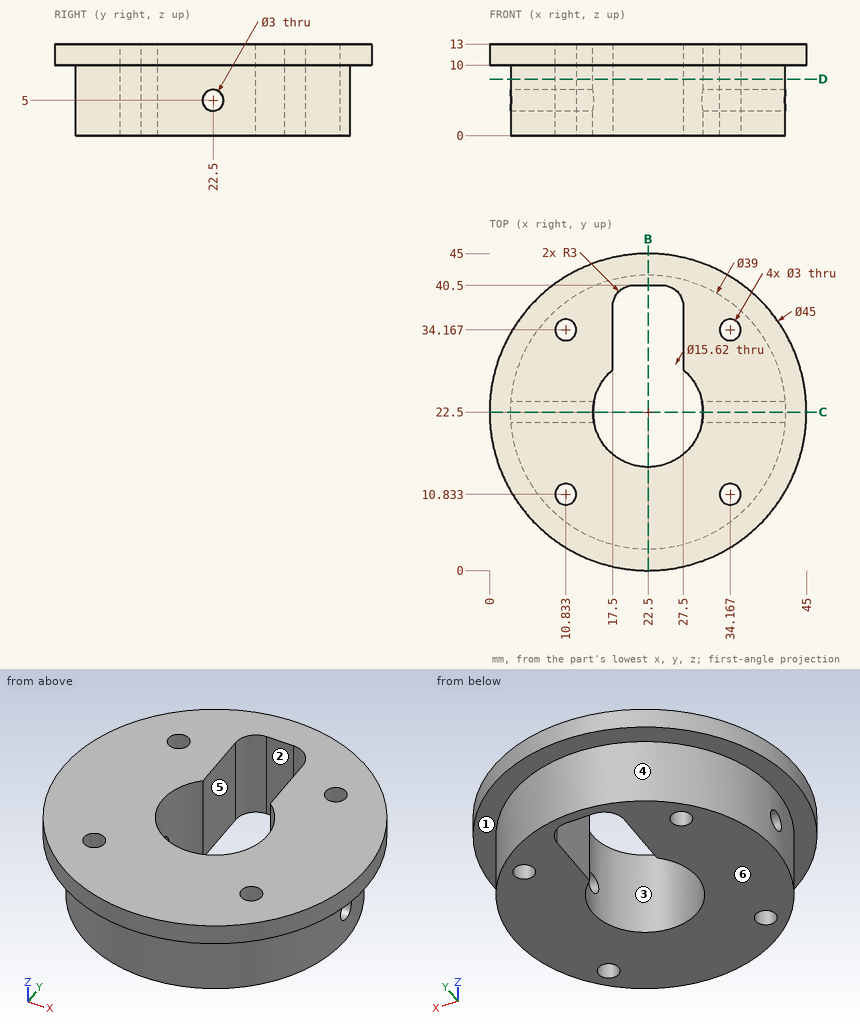
Can you work these out from the drawing? Everything is in mm from the part's minimum corner. A direction names the side the tool comes from. Give positions to 0.01 mm unless a question says otherwise; leave off trailing zeros. Order: outer loops, then holes, each group sorted by start corner. A loop starts at its lowest first (then second) coordinate and runs counter-clockwise, first axis right, second up. Notation, with made-up numbers: M 34,71.5 L 92,71.5 A26 ccw 92,99.5 Z; hole C -30.5,28 d8. An arc over 180 degrees is marked long. Use a Markdown table: item, result. Add a question column.
Item 1: If I drill on L1, parallel to Y at x = 35.5, z = 5.5 (1 decimal); L2, parallel to X at y = 22.5, z = 9; L3, parallel to X at y = 35.5, z = 6.5 (1 decimal), over which ranges is the centre line in solid material (lowest first)? Write a range as [from, to].
Item 2: Suppose I cut it at B-B (x = 22.5). List the corners of the cut face in (y, z) for me.
Item 3: For the marked faces 5 and 6, which set-ups out of +Z, -Z, +X, -X, +Y, -Y let a thin tool reach every point of the face, with its end or its side?
Item 4: We'd pull the mould along X, two halves only. Please class the marked faces 1, 2, 3 and 4: +X half, -X half, draft (parallel to the pull), parting line (faces both ways), or undercut.
Item 5: Suppose I cut it at D-D (z = 8). List the corners of the cut face in (x, y) for me, then the cut area to 3 significant figures.
Item 6: Suppose I cut it at C-C (y = 22.5). List the corners of the cut face in (x, z) for me, then the cut area to 3 significant figures.
Item 7: Will these pins go through, and if not, where does the flat tip stop? pin 1 (2.5 mm diameter, centred on y = 22.5, z = 5, fed in from +X); pin 2 (6 mm diameter, centred on x = 12, z = 6.5, fed in from -Y); pin 3 (4 mm diameter, centred on x = 21, z = 2, fed in from +Y); pin 4 (4.5 mm diameter, centred on y = 34.5, z = 8.5, fed in from +X).
Answer sheet:
| question | item | result |
|---|---|---|
| 1 | L1 | y = [8, 10.1], [11.5, 21.1], [23.9, 33.5], [34.9, 37] |
| 1 | L2 | x = [3, 14.69], [30.31, 42] |
| 1 | L3 | x = [8, 10.1], [11.5, 17.5], [27.5, 33.5], [34.9, 37] |
| 2 | outline | M 0,10 L 3,10 L 3,0 L 14.69,0 L 14.69,13 L 0,13 Z; M 40.5,0 L 42,0 L 42,10 L 45,10 L 45,13 L 40.5,13 Z |
| 3 | face 5 | +Z, -Z |
| 3 | face 6 | -Z, +X, -X, +Y, -Y |
| 4 | face 1 | draft |
| 4 | face 2 | undercut |
| 4 | face 3 | undercut |
| 4 | face 4 | parting line |
| 5 | outline | C 22.5,22.5 d39; hole C 10.83,10.83 d3; hole C 10.83,34.17 d3; hole M 17.5,28.5 A7.81 ccw long 27.5,28.5 L 27.5,37.5 A3 ccw 24.5,40.5 L 20.5,40.5 A3 ccw 17.5,37.5 Z; hole C 34.17,10.83 d3; hole C 34.17,34.17 d3 |
| 5 | area | 871 mm² |
| 6 | outline | M 0,10 L 3,10 L 3,6.5 L 14.69,6.5 L 14.69,13 L 0,13 Z; M 3,0 L 14.69,0 L 14.69,3.5 L 3,3.5 Z; M 30.31,0 L 42,0 L 42,3.5 L 30.31,3.5 Z; M 30.31,6.5 L 42,6.5 L 42,10 L 45,10 L 45,13 L 30.31,13 Z |
| 6 | area | 252 mm² |
| 7 | pin 1 | passes through |
| 7 | pin 2 | stops at y = 4.5 |
| 7 | pin 3 | stops at y = 42 |
| 7 | pin 4 | stops at x = 42.49 |
